from build123d import *

# Parameters (mm, degrees)
SKETCH6_R           = 0.215
EXTRUDE2_DEPTH      = 6.5
CUT_EXTRUDE1_DEPTH  = 8.611175993
FILLET1_R           = 0.2
FILLET2_R           = 0.1
SKETCH6_3_R         = 0.265
SKETCH6_3_R_2       = 0.215
BOSS_EXTRUDE2_DEPTH = 0.05


with BuildPart() as part:
    # Sketch4 → Revolve2 (revolve)
    with BuildSketch(Plane.XY, mode=Mode.PRIVATE) as revolve2_sk:
        with BuildLine():
            Line((0, 0), (0, 0.7))
            Line((0, 0.7), (-0.75, 0.7))
            Line((-0.75, 0.7), (-0.75, 0.8))
            Line((-0.75, 0.8), (-1, 0.8))
            Line((-1, 0.8), (-1, 1.775))
            Line((-1, 1.775), (0.75, 1.775))
            ThreePointArc((0.75, 1.775), (0.926776695, 1.848223305), (1, 2.025))
            Line((1, 2.025), (1, 2.1))
            Line((1, 2.1), (1.3, 2.1))
            Line((1.3, 2.1), (1.3, 2.8))
            Line((1.3, 2.8), (2.5, 2.8))
            Line((2.5, 2.8), (2.5, 0))
            Line((2.5, 0), (0, 0))
        make_face()
    revolve(revolve2_sk.sketch.rotate(Axis((-2.49171246, 0, 0), (1, 0, 0)), 90), axis=Axis((-2.49171246, 0, 0), (1, 0, 0)))

    # Sketch6 → Extrude2 (add)
    with BuildSketch(Plane(origin=(2.5, 0, 0), x_dir=(0, 0, -1), z_dir=(1, 0, 0))):
        with Locations(Location((0, -1, 0), (0, 0, 180))):
            Circle(SKETCH6_R)
        with Locations(Location((-1, 0, 0), (0, 0, 180))):
            Circle(SKETCH6_R)
        with Locations(Location((1, 0, 0), (0, 0, 180))):
            Circle(SKETCH6_R)
        with Locations(Location((0, 1, 0), (0, 0, 180))):
            Circle(SKETCH6_R)
    extrude(amount=EXTRUDE2_DEPTH)

    # Sketch8 → Cut-Extrude1 (cut, through all)
    with BuildSketch(Plane(origin=(2.5, 0, 0), x_dir=(0, 0, -1), z_dir=(1, 0, 0))):
        with BuildLine():
            Line((-2.4, 0), (-2.774801575, 0.374801575))
            ThreePointArc((-2.774801575, 0.374801575), (-2.8, 0), (-2.774801575, -0.374801575))
            Line((-2.774801575, -0.374801575), (-2.4, 0))
        make_face()
        with BuildLine():
            Line((2.774801575, 0.374801575), (2.4, 0))
            Line((2.4, 0), (2.774801575, -0.374801575))
            ThreePointArc((2.774801575, -0.374801575), (2.793693291, -0.187823841), (2.8, 0))
            ThreePointArc((2.8, 0), (2.793693291, 0.187823841), (2.774801575, 0.374801575))
        make_face()
        with BuildLine():
            ThreePointArc((-0.5, -2.754995463), (0, -2.8), (0.5, -2.754995463))
            Line((0.5, -2.754995463), (0.5, -2.4))
            Line((0.5, -2.4), (-0.5, -2.4))
            Line((-0.5, -2.4), (-0.5, -2.754995463))
        make_face()
    extrude(amount=-CUT_EXTRUDE1_DEPTH, mode=Mode.SUBTRACT)

    # Fillet1
    fillet1_edges = [part.edges().sort_by_distance(p)[0] for p in [
        (-1, 0, -1.775),
    ]]
    fillet(fillet1_edges, radius=FILLET1_R)

    # Fillet2
    fillet2_edges = [part.edges().sort_by_distance(p)[0] for p in [
        (1.3, 2.8, 0),
        (1.3, -1.934576937, -2.02420653),
        (1.3, -1.934576937, 2.02420653),
    ]]
    fillet(fillet2_edges, radius=FILLET2_R)

    # Sketch6<3> → Boss-Extrude2 (add)
    with BuildSketch(Plane(origin=(2.5, 0, 0), x_dir=(0, 0, -1), z_dir=(1, 0, 0))):
        with Locations(Location((0, -1, 0), (0, 0, 180))):
            Circle(SKETCH6_3_R)
        with Locations((0, -1)):
            Circle(SKETCH6_3_R_2, mode=Mode.SUBTRACT)
    extrude(amount=BOSS_EXTRUDE2_DEPTH)


solid = part.part
Can you work these out from the model? Positions are in its coordinate system, mm. A direction names the side the tool comes from. Coordinates: 2 decimals unless noted, no trailing zeros. Order: outer loops, then holes, each group sorted by start corner. A loop starts at its lowest first (then second) coordinate and runs counter-clockwise, first axis right, second up. Notation, with made-up numbers: (48.25, 38.25) -> (95.25, 38.25) arc R20 ccw to (95.25, 61.25) -> close; hole circle Ø5 at (-4.5, 20.25). An arc over 180 degrees is marked (long way). Use one line per item in the form item = value.
Q1. Imagine slicing it at A-A, the plane x = 6.5. List the corners of the cut face in (y, z) for me (3 decimals), then the cut area to 3 significant figures.
From the geometry:
outline = circle Ø0.43 at (-1, 0); circle Ø0.43 at (0, -1); circle Ø0.43 at (0, 1); circle Ø0.43 at (1, 0)
area = 0.581 mm²
Q2. Which directions (+Z, -Z, +X, -X, +Y, -Y) give clear straight access to the entire face, cutting with the end or side of a thin tool? Please do faces 1 (the face through (2, -2.4, 0)), 2 (the face through (-0.4, 0, -0.7)), 3 (the face through (2.5, 0, 0)).
From the geometry:
face_1 = +X, -X, -Y
face_2 = -X
face_3 = +X
Q3. We'd pull the mould along Y, two halves only. Please class faces 4 (the face through (0, 0, 0)), 5 (the face through (1.15, -0.09, -2.1)), 6 (the face through (-1, 0, 1)), 7 (the face through (1.96, -1.95, -2.01)): released by +Y, released by -Y, zero draft, split by the parting line, or undercut.
From the geometry:
face_4 = undercut
face_5 = split by the parting line
face_6 = zero draft
face_7 = released by -Y
Q4. I need wall thicknesses on L1, parallel to Y at x = -0.25, z = 0 (3 decimals); L2, parallel to X at y = -1.1, z = -1.85; L3, parallel to X at y = -0.2, z = -0.4. Which ranges of each line are inside material? Lowest first, please.
From the geometry:
L1 = -1.775 to -0.7, 0.7 to 1.775
L2 = 1.3 to 2.5
L3 = 0 to 2.5
Q5. Will these pins go through, and if not, where does the flat tip stop? P1, Ø0.5, axis at x = 2, z = 0, coming from the -Y side; P2, Ø0.5, axis at y = -0.5, z = 0, coming from the -X side; P3, Ø1, axis at y = 2, z = -2, coming from the +X side.
From the geometry:
P1 = -2.4
P2 = -0.75
P3 = 2.5
